```python
from build123d import *

# Parameters (mm, degrees)
EXTRUDE007_DEPTH = 1
BOX003_W         = 8
BOX003_H         = 8
BOX003_DEPTH     = 1


with BuildPart() as snapsnapextrude:
    # Sketch006 (on Face6 of Box003) → Extrude007 (new body)
    with BuildSketch(Plane(origin=(30.86, 17.4167, 1), x_dir=(1, 0, 0), z_dir=(0, 0, 1))):
        with BuildLine():
            Line((5.5, 9), (5.5, 8))
            Line((4.771508, 8), (5.5, 8))
            Line((5.007358, 8.23585), (4.771508, 8))
            Line((5.007358, 9.571194), (5.007358, 8.23585))
            Line((5.007358, 9.571194), (5.5, 9.571194))
            ThreePointArc((6.071194, 9), (5.903895, 9.403895), (5.5, 9.571194))
            Line((5.5, 9), (6.071194, 9))
        make_face()
        with BuildLine():
            Line((2.5, 8), (2.5, 9))
            Line((1.928806, 9), (2.5, 9))
            ThreePointArc((2.5, 9.571194), (2.096105, 9.403895), (1.928806, 9))
            Line((2.5, 9.571194), (2.992642, 9.571194))
            Line((2.992642, 8.23585), (2.992642, 9.571194))
            Line((2.992642, 8.23585), (3.228492, 8))
            Line((2.5, 8), (3.228492, 8))
        make_face()
    extrude(amount=-EXTRUDE007_DEPTH)


with BuildPart() as snapsnap:
    # Box003 → Box003 (new body)
    with BuildSketch(Plane(origin=(30.86, 17.4167, 0), x_dir=(1, 0, 0), z_dir=(0, 0, 1))):
        with Locations((4, 4)):
            Rectangle(BOX003_W, BOX003_H)
    extrude(amount=BOX003_DEPTH)

    # Fusion: union snapSnapExtrude
    add(snapsnapextrude.part)


solid = snapsnap.part
```
Verification items for the finished model (mm, model axes). A direction names the side the tool comes from. Give positions to 0.01 mm unless a question says otherwise; leave off trailing zeros. Order: outer loops, then holes, each group sorted by start corner. A loop starts at its lowest first (then second) coordinate and runs counter-clockwise, first axis right, second up. Notation, with made-up numbers: (-40, -9) - (-30, -9) arc R20 ccw to (-30, 19) - close; hole circle Ø9 at (-12, -16.5). An arc over 180 degrees is marked (long way). Answer as CSV lines item,"result". Start each with the question number.
Item 1: Section check C-C, the plane x = 37.5. Record the boundary of the cut face in (y, z), plus the area to 3 significant figures.
Item 2: Gauge pin test, flat ends, axial feed: pin 1 (0.5 mm diameter, centred on x = 38, z = 0.5, fed in from +Y); pin 2 (0.5 mm diameter, centred on y = 26, z = 0.5, fed in from +X); pin 3 (0.5 mm diameter, centred on y = 26.5, z = 0.5, fed in from -X). Record the tip position at first contact, or that the pin passes through.
Item 3: Access from +Z, -Z, +X, -X, +Y, -Y to the whole of each face (thin tool, end or side, straight path). Record for faces 1 (the face through (33.853, 26.3, 0.5)), 2 (the face through (35, 21, 0)), 3 (the face through (34.8, 17.417, 0.5)), 4 (the face through (36.36, 25.9, 0.5)), 5 (the face through (32.1, 25.417, 0.5)).
Item 4: Material ranges on L1, parallel to Y at x = 34.5, z = 0.7; L2, parallel to Y at x = 33.25, z = 0.15; L3, parallel to X at y = 26.5, z = 0.9, recorded low to high.
Item 5: Mould release check, pull along X, two halves, no side actions. Record for faces 6 (the face through (34.8, 25.417, 0.5)), 7 (the face through (37.6, 25.417, 0.5)), 8 (the face through (38.86, 21.4, 0.5)): released by +X, released by -X, zero draft, split by the parting line, or undercut.
Item 6: Section check B-B, the plane y = 26.25. Record the boundary of the cut face in (x, z).
Item 7: Section check A-A, the plane z = 0.75. Record the boundary of the cut face in (x, y), plus the area to 3 significant figures.
Filled in:
1,outline,"(17.42, 0) - (25.42, 0) - (25.42, 1) - (17.42, 1) - close"
1,area,"8.00 mm^2"
2,pin 1,"y = 25.42"
2,pin 2,"x = 36.36"
2,pin 3,"x = 32.79"
3,face 1,"+Z, -Z, +Y"
3,face 2,"-Z, +X, -X, +Y, -Y"
3,face 3,"+Z, -Z, +X, -X, -Y"
3,face 4,"+Z, -Z, +X"
3,face 5,"+Z, -Z, -X"
4,L1,"17.42 to 25.42"
4,L2,"17.42 to 25.42, 26.42 to 26.98"
4,L3,"32.79 to 33.85, 35.87 to 36.93"
5,face 6,"undercut"
5,face 7,"zero draft"
5,face 8,"released by +X"
6,outline,"(33.36, 0) - (33.85, 0) - (33.85, 1) - (33.36, 1) - close; (35.87, 0) - (36.36, 0) - (36.36, 1) - (35.87, 1) - close"
7,outline,"(30.86, 17.42) - (38.86, 17.42) - (38.86, 25.42) - (36.36, 25.42) - (36.36, 26.42) - (36.93, 26.42) arc R0.57 ccw to (36.36, 26.99) - (35.87, 26.99) - (35.87, 25.65) - (35.63, 25.42) - (34.09, 25.42) - (33.85, 25.65) - (33.85, 26.99) - (33.36, 26.99) arc R0.57 ccw to (32.79, 26.42) - (33.36, 26.42) - (33.36, 25.42) - (30.86, 25.42) - close"
7,area,"66.1 mm^2"
